Can you work these out from the model? Positions are in its coordinate system, mm. A direction names the side the tool comes from. Give positions to 0.01 mm unless a question says otherwise; leave off trailing zeros. Order: outer loops, then holes, each group sorted by start corner. A loop starts at its lowest first (then second) coordinate and runs counter-clockwise, first axis right, second up. Notation, with made-up numbers: (60.5, 26) - (114.5, 26) arc R6 ccw to (114.5, 33) - close; hole circle Ø8 at (-20.75, 86.25). An arc over 180 degrees is marked (long way). Write each question's results on one line, items separated by ' | '. Start each with the question number.
from build123d import *

# Parameters (mm, degrees)
F1_DEPTH = 30
F3_DEPTH = 32.501


with BuildPart() as f1:
    # F0 (on Top) → F1 (new body)
    with BuildSketch(Plane.XY):
        Polygon((0, 7), (0, 0), (60, 0), (60, 32.5), (0, 32.5), (0, 25.5), (20, 25.5), (20, 7), align=None)
    extrude(amount=F1_DEPTH)

    # F2 (on face) → F3 (cut, through all)
    with BuildSketch(Plane.XZ):
        with BuildLine():
            ThreePointArc((30, 15), (40, 5), (50, 15))
            ThreePointArc((50, 15), (40, 25), (30, 15))
        make_face()
        with BuildLine():
            ThreePointArc((30, 15), (40, 25), (50, 15))
            Line((50, 15), (50, 30))
            Line((50, 30), (30, 30))
            Line((30, 30), (30, 15))
        make_face()
    extrude(amount=-F3_DEPTH, mode=Mode.SUBTRACT)

    # F5 (on plane+point) → F6 (revolve, cut)
    with BuildSketch(Plane.XY.offset(15)):
        with BuildLine():
            ThreePointArc((40, 15), (52.3743686708, 20.1256313292), (57.5, 32.5))
            Line((57.5, 32.5), (40, 32.5))
            Line((40, 32.5), (40, 15))
        make_face()
    revolve(axis=Axis((40, 23.75, 15), (0, -1, 0)), mode=Mode.SUBTRACT)


solid = f1.part
Q1. Which directions (+Z, -Z, +X, -X, +Y, -Y) give clear straight access to the entire face, cutting with the end or side of a thin tool? Please do faces 1 (the flat face through (21, 16, 30)), 2 (the flat face through (10, 7, 15)), 3 (the flat face through (50, 12, 22)).
Q2. If I drill on probe 1 along X at (y, z) = (8.5, 28); probe 2 along X at (y, z) = (4.5, 18.5); probe 3 along Y at (x, z) = (15.5, 9), over which ranges is the centre line in solid material (lowest first)? Write a range as from..to.
Q3. If we section it at C-C (y = 12): Please give me the cut outline in (x, z).
Q4. Thinking about a two-plate mould opening in X: for faces 4 (the flat face through (30, 12, 23)), 5 (the flat face through (10, 25.5, 15)), 6 (the flat face through (20, 16, 15)), which applies, released by +X, released by -X, zero draft, split by the parting line, or undercut?
Q5. If we section it at D-D (z = 6.5): Please give me the cut outline in (x, y).
Q6. If we section it at A-A (x = 14.5): Please give me the cut outline in (y, z), plus the area to 3 significant figures.
Q7. Will these pins go through, and if not, where does the flat tip stop? P1, Ø5, axis at x = 36, y = 15.5, coming from the +Z side; P2, Ø5, axis at y = 21.5, z = 7.5, coming from the -X side; P3, Ø2, axis at x = 41.5, y = 8, coming from the +Z side.
Q8. If we section it at B-B (z = 23): Please give me the cut outline in (x, y).
Findings below:
1) face 1: +Z, +X, -X, +Y, -Y | face 2: +Z, -Z, -X | face 3: +Z, +Y, -Y
2) probe 1: x = 20..30, 50..60 | probe 2: x = 0..30, 50..60 | probe 3: y = 0..7, 25.5..32.5
3) outline: (20, 0) - (60, 0) - (60, 30) - (50, 30) - (50, 15) arc R10 cw to (30, 15) - (30, 30) - (20, 30) - close
4) face 4: undercut | face 5: zero draft | face 6: released by -X
5) outline: (0, 0) - (34.73, 0) - (34.73, 18.14) arc R15.3 cw to (24.7, 32.5) - (0, 32.5) - (0, 25.5) - (20, 25.5) - (20, 7) - (0, 7) - close; (45.27, 0) - (60, 0) - (60, 32.5) - (55.3, 32.5) arc R15.3 cw to (45.27, 18.14) - close
6) outline: (0, 0) - (7, 0) - (7, 30) - (0, 30) - close; (25.5, 0) - (32.5, 0) - (32.5, 30) - (25.5, 30) - close | area: 420 mm2
7) P1: stops at z = 7.4 | P2: stops at x = 20 | P3: stops at z = 5.32
8) outline: (0, 0) - (30, 0) - (30, 20.57) arc R15.56 cw to (24.44, 32.5) - (0, 32.5) - (0, 25.5) - (20, 25.5) - (20, 7) - (0, 7) - close; (50, 0) - (60, 0) - (60, 32.5) - (55.56, 32.5) arc R15.56 cw to (50, 20.57) - close
